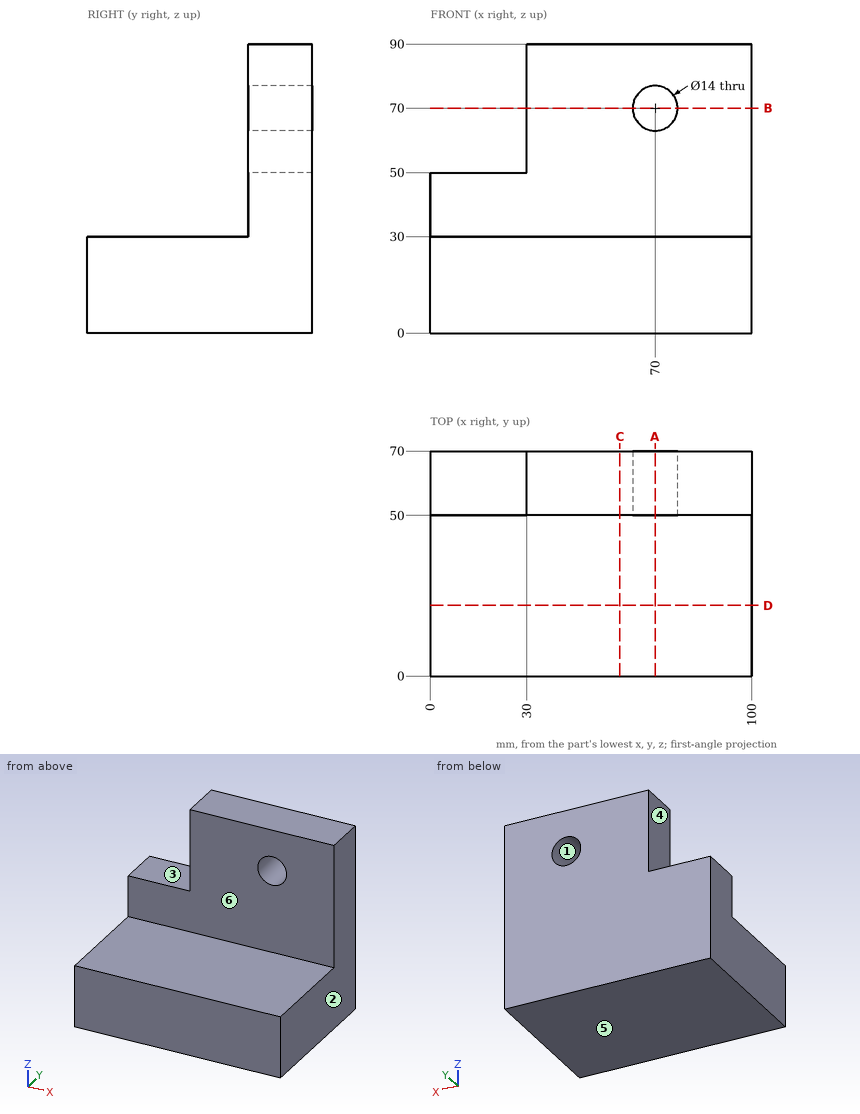
Study the drawing (mm; zero at the part's minimum x, y, z) and answer. A direction names the side the tool comes from. Round coordinates to 2 decimals unless told otherwise and drop trailing zeros. Loops run counter-clockwise (first coordinate to the right, second up) from the corner with the lowest first, then second, coordinate; pieces in that order, holes last. Notation, with made-up numbers: (-37, -38.75) -> (-3, -38.75) arc R18 cw to (-3, -29.75) -> close; hole circle Ø3 at (0, 44.25). An arc over 180 degrees is marked (long way). One line per item, written item: value.
1) A cutting plane is placed at C-C (x = 59). Determine the outline of the cut face in (y, z), and give its area (3 significant figures).
Answer list:
outline: (0, 0) -> (70, 0) -> (70, 90) -> (50, 90) -> (50, 30) -> (0, 30) -> close
area: 3,300 mm²
2) Consider L1, parallel to Z at x = 70, y = 63; L2, parallel to Z at x = 32, y = 41.5; L3, parallel to Y at x = 66, z = 38. Determine where each line is inside the solid, lowest interval first. Write a range as [from, to].
Answer list:
L1: z = [0, 63], [77, 90]
L2: z = [0, 30]
L3: y = [50, 70]
3) A cutting plane is placed at B-B (z = 70). Determine the outline of the cut face in (x, y).
Answer list:
outline: (30, 50) -> (63, 50) -> (63, 70) -> (30, 70) -> close; (77, 50) -> (100, 50) -> (100, 70) -> (77, 70) -> close
4) A cutting plane is placed at A-A (x = 70). Determine the outline of the cut face in (y, z).
Answer list:
outline: (0, 0) -> (70, 0) -> (70, 63) -> (50, 63) -> (50, 30) -> (0, 30) -> close; (50, 77) -> (70, 77) -> (70, 90) -> (50, 90) -> close
5) A cutting plane is placed at D-D (y = 22). Determine the outline of the cut face in (x, z).
Answer list:
outline: (0, 0) -> (100, 0) -> (100, 30) -> (0, 30) -> close
6) For the marked faces 4, 5 and 6, determine the directions among +Z, -Z, +X, -X, +Y, -Y from which every point of the face is accessible in a straight line to the end or side of a thin tool.
Answer list:
face 4: +Z, -X, +Y, -Y
face 5: -Z, +X, -X, +Y, -Y
face 6: +Z, +X, -X, -Y
7) Flat-ended cylindrical pins translate along their axes: P1, Ø3, axis at x = 64.5, y = 36, coming from the +Z side; P2, Ø6, axis at x = 19, y = 59.5, coming from the +Z side; P3, Ø10, axis at y = 63.5, z = 67.5, coming from the -X side. Find the tip coordinate at first contact, or state that the pin passes through.
Answer list:
P1: stops at z = 30
P2: stops at z = 50
P3: stops at x = 30
8) The mould has two halves that part along X. Classify the marked faces 1, 2 and 3: pulls with the +X half, pulls with the -X half, needs draft (parallel to the pull), parting line crosses it, or undercut.
Answer list:
face 1: undercut
face 2: pulls with the +X half
face 3: needs draft
